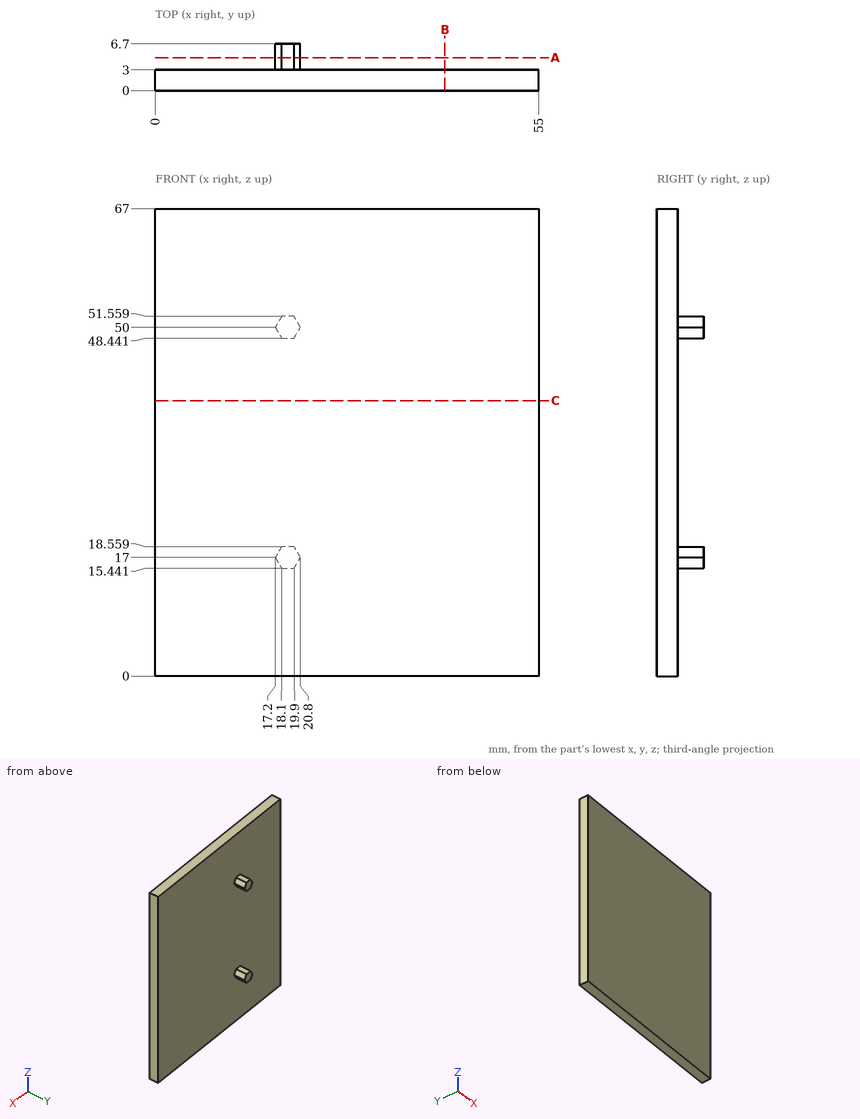
Study the drawing (mm; zero at the part's minimum x, y, z) and answer. Give positions to 0.01 mm unless a question says otherwise; leave off trailing zeros. Loops run counter-clockwise (first coordinate to the right, second up) from the corner with the lowest first, then second, coordinate; pieces in that order, holes last. Notation, with made-up numbers: M 27.5,72 L 36.5,72 A29 ccw 36.5,94 Z; hole C 6,-34.5 d3. An arc over 180 degrees is marked long. Answer as CSV lines item,"result".
Item 1: Straight lines are drawn through the part: line 1 along Y through (x, z) = (42, 40); line 2 along Z through (x, y) = (20, 5.5) (1 decimal). For each, find the intervals that lie inside material, in ascending order. Write a range as [from, to].
Values follow:
line 1,"y = [0, 3]"
line 2,"z = [15.6, 18.4], [48.6, 51.4]"
Item 2: Given pin 1 Ø0.5 at (x, y) = (18.5, 4) entering from -Z; pin 2 Ø3 at (x, y) = (26, 5) entering from -Z; pin 3 Ø1.5 at (x, z) = (46, 45) entering from +Y; pin 4 Ø0.5 at (x, y) = (19, 4.5) entering from +Z, each flat-ended and moving along its own axis, determine where each tip first touches the part or whether it passes through.
Values follow:
pin 1,"stops at z = 15.44"
pin 2,"passes through"
pin 3,"stops at y = 3"
pin 4,"stops at z = 51.56"
Item 3: The part is cut by section C-C (z = 39.5). Give the vertices of the cut face in (x, y).
Values follow:
outline,"M 0,0 L 55,0 L 55,3 L 0,3 Z"
Item 4: The part is cut by section B-B (x = 41.5). Give the vertices of the cut face in (y, z), and give its area (3 significant figures).
Values follow:
outline,"M 0,0 L 3,0 L 3,67 L 0,67 Z"
area,"201 mm^2"
Item 5: The part is cut by section A-A (y = 4.75). Give the vertices of the cut face in (x, z), and give its area (3 significant figures).
Values follow:
outline,"M 17.2,17 L 18.1,15.44 L 19.9,15.44 L 20.8,17 L 19.9,18.56 L 18.1,18.56 Z; M 17.2,50 L 18.1,48.44 L 19.9,48.44 L 20.8,50 L 19.9,51.56 L 18.1,51.56 Z"
area,"16.8 mm^2"
